Could you check a few things on this drawing? It's one solid part, dimensions in mm from its lowest x, y, z. A direction names the side the tool comes from. Coordinates: 2 decimals unless noted, no trailing zeros. Write each loop counter-clockwise with the first axis right and the second up, starting at its lowest first coordinate (ties: lowest second). Pieces come first, ordered by that corner, then holes.
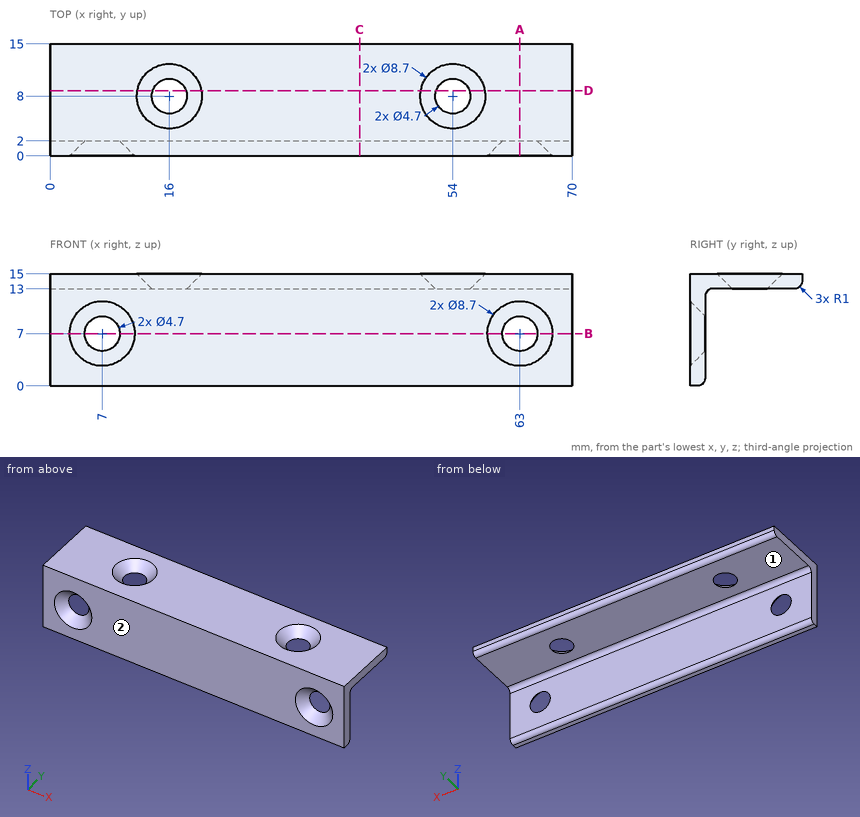
1) On a 3-axis mill with a long thin cutter (end or side, diameter ignored), from which of +Z, -Z, +X, -X, +Y, -Y can I reach the whole of each face in a straight line? I mean the marked faces 1 and 2. Say none if no direction works.
Values follow:
face 1: -Z, +X, -X, +Y
face 2: +Z, -Z, +X, -X, -Y
2) Imagine slicing it at A-A on x = 63. Please give me the cut outline in (y, z).
Values follow:
outline: (0, 0) - (1, 0) arc R1 ccw to (2, 1) - (2, 4.65) - (0, 2.65) - close; (0, 11.35) - (2, 9.35) - (2, 12) arc R1 cw to (3, 13) - (14, 13) arc R1 ccw to (15, 14) - (15, 15) - (0, 15) - close
3) Imagine slicing it at D-D on y = 8.75. Count the separate pieces of the cut face and the enclosed holes in it, then the cut area to 3 significant figures.
Values follow:
separate pieces: 3
enclosed holes: 0
area: 114 mm2
4) Imagine slicing it at C-C on x = 41.5. Please give me the cut outline in (y, z).
Values follow:
outline: (0, 0) - (1, 0) arc R1 ccw to (2, 1) - (2, 12) arc R1 cw to (3, 13) - (14, 13) arc R1 ccw to (15, 14) - (15, 15) - (0, 15) - close
5) Imagine slicing it at B-B on z = 7. Please give me the cut outline in (x, y), then the cut area to 3 significant figures.
Values follow:
outline: (0, 0) - (2.65, 0) - (4.65, 2) - (0, 2) - close; (9.35, 2) - (11.35, 0) - (58.65, 0) - (60.65, 2) - close; (65.35, 2) - (67.35, 0) - (70, 0) - (70, 2) - close
area: 113 mm2
6) I need wall thicknesses on probe 1 along Y at (x, z) = (47, 11.75); probe 2 along Z at (x, y) = (43, 6.5); probe 3 along Y at (x, z) = (17, 14.25). Which ranges of each line are inside material? Lowest first, please.
Values follow:
probe 1: y = 0 to 2
probe 2: z = 13 to 15
probe 3: y = 0 to 4.54, 11.46 to 15
7) Will these pins go through, and if not, where does the flat tip stop? pin 1 (6 mm diameter, centred on x = 19.5, z = 8, fed in from -Y); pin 2 (9 mm diameter, centred on x = 39, y = 11, fed in from -Z); pin 3 (4 mm diameter, centred on x = 18, z = 6, fed in from +Y).
Values follow:
pin 1: stops at y = 0
pin 2: stops at z = 13
pin 3: stops at y = 2
